The model under review builds one solid part; all positions refer to its coordinate system, in mm. Face numbers are marked on the shaded views. A direction names the side the tool comes from. Coordinates: 2 decimals unless noted, no trailing zeros. Order: outer loops, then holes, each group sorted by start corner. A loop starts at its lowest first (then second) coordinate and runs counter-clockwise, first axis right, second up. Notation, with made-up numbers: M 46.25,26 L 105.25,26 A13 ccw 105.25,33 Z; hole C 8,4 d7. An arc over 180 degrees is marked long. Answer as CSV lines item,"result". Start each with the question number.
Q1. Consider section C-C on z = 15. Write out the cut boundary in (x, y).
Q2. Consider section B-B on x = -29. Write out the cut boundary in (y, z), and give its area (3 significant figures).
Q3. Wall thickness on L1, parallel to Z at x = -2.95, y = -2.5; L2, parallel to Y at x = -29, z = 0; L3, parallel to X at y = -3, z = -17.5: over which ranges is each line inside the solid? List them lowest first. Write a range as [from, to].
Q4. Machinability: for the marked faces 4, 5 and 6, which of the approach directions +Z, -Z, +X, -X, +Y, -Y give a long, thin tool a straight path to every point of the face, cutting with its end or side? Answer none if there is none.
Q5. The part is to be moulded in two halves that separate along Y. For the marked faces 1, 2 and 3, say which applies: +Y half, -Y half, draft (parallel to the pull), parting line (faces both ways), or undercut.
Q6. Consider section A-A on z = -4.5. Write out the cut boundary in (x, y).
Q7. For P1, Ø0.9, axis at y = -6.5, z = -21, coming from the -X side; P2, Ø5, axis at x = -28.5, y = -3.5, coming from the -Z side; P3, Ø1.5, axis at x = -5.5, y = -5.5, coming from the -Z side; P4, Ø10.5, axis at y = -2.5, z = -15, coming from the +X side, all flat-tipped, find the tip position at first contact; note any pin that passes through.
Q8. Consider section D-D on y = -2.5. State how many separate pieces and enclosed holes the cut face has, and give its area (3 significant figures).
from build123d import *

# Parameters (mm, degrees)
F0_W          = 36.5
F0_H          = 20
F0_R          = 4.75
F1_DEPTH      = 5
F1_DEPTH_BACK = 5
F2_SIZE       = 2
F3_W          = 20
F3_H          = 46
F3_R          = 4
F4_DEPTH      = 4
F5_T4_DEPTH   = 20
F5_S5_R       = 4
F5_T6_DEPTH   = 16
F5_T10_DEPTH  = 20
F5_S11_R      = 4
F5_T12_DEPTH  = 16
F3_R_2        = 2.15
F6_DEPTH      = 4
F7_R          = 5
F8_R          = 5


# Not quite as in the source:
# - a fillet or chamfer that OpenCascade refuses, or shapes differently, is made with other operations: its cross-section is extruded or revolved along the edge and cut away or added


with BuildPart() as f1:
    # F0 (on Top) → F1 (new body, two sides)
    with BuildSketch(Plane.XY) as f1_sk:
        with Locations((-18.25, -2.5)):
            Rectangle(F0_W, F0_H)
        with Locations((-29, 0)):
            Circle(F0_R, mode=Mode.SUBTRACT)
    extrude(amount=F1_DEPTH)
    extrude(f1_sk.sketch, amount=-F1_DEPTH_BACK)

    # F2
    f2_edges = [f1.edges().sort_by_distance(p)[0] for p in [
        (-33.75, 0, 5),
        (-33.75, 0, -5),
    ]]
    chamfer(f2_edges, length=F2_SIZE)

    # F3 (on Right) → F4 (join)
    with BuildSketch(Plane.YZ):
        with Locations((-2.5, 0)):
            Rectangle(F3_W, F3_H)
        with Locations((-2.5, -15)):
            Circle(F3_R, mode=Mode.SUBTRACT)
        with Locations((-2.5, 15)):
            Circle(F3_R, mode=Mode.SUBTRACT)
    extrude(amount=-F4_DEPTH)

    # F5: fillet of radius 15 on 2 edges, made by hand


with BuildPart() as f5_tool2:
    # F5_s3 → F5_t4 (new body)
    with BuildSketch(Plane.XZ.offset(12.5)):
        with BuildLine():
            ThreePointArc((-19, 5), (-8.3933982822, 9.3933982822), (-4, 20))
            Line((-4, 20), (-4, 5))
            Line((-4, 5), (-19, 5))
        make_face()
    extrude(amount=-F5_T4_DEPTH)

    # F5_s5 → F5_t6 (cut, symmetric)
    with BuildSketch(Plane.YZ.offset(-11.5)):
        with Locations((-2.5, 15)):
            Circle(F5_S5_R)
    extrude(amount=F5_T6_DEPTH, both=True, mode=Mode.SUBTRACT)


with BuildPart() as f1_1:
    add(f1.part)

    # F5_t1: union F5_tool2
    add(f5_tool2.part)


with BuildPart() as f5_tool8:
    # F5_s9 → F5_t10 (new body)
    with BuildSketch(Plane.XZ.offset(12.5)):
        with BuildLine():
            ThreePointArc((-4, -20), (-8.3933982822, -9.3933982822), (-19, -5))
            Line((-19, -5), (-4, -5))
            Line((-4, -5), (-4, -20))
        make_face()
    extrude(amount=-F5_T10_DEPTH)

    # F5_s11 → F5_t12 (cut, symmetric)
    with BuildSketch(Plane.YZ.offset(-11.5)):
        with Locations((-2.5, -15)):
            Circle(F5_S11_R)
    extrude(amount=F5_T12_DEPTH, both=True, mode=Mode.SUBTRACT)


with BuildPart() as f1_2:
    add(f1_1.part)

    # F5_t7: union F5_tool8
    add(f5_tool8.part)

    # F3 (on Right) → F6 (join)
    with BuildSketch(Plane.YZ):
        with Locations((-2.5, 15)):
            Circle(F3_R)
        with Locations((-2.5, 15)):
            Circle(F3_R_2, mode=Mode.SUBTRACT)
        with Locations((-2.5, -15)):
            Circle(F3_R)
        with Locations((-2.5, -15)):
            Circle(F3_R_2, mode=Mode.SUBTRACT)
    extrude(amount=-F6_DEPTH)

    # F7
    f7_edges = [f1_2.edges().sort_by_distance(p)[0] for p in [
        (-2, -12.5, -23),
        (-2, -12.5, 23),
        (-2, 7.5, -23),
        (-2, 7.5, 23),
    ]]
    fillet(f7_edges, radius=F7_R)

    # F8
    f8_edges = [f1_2.edges().sort_by_distance(p)[0] for p in [
        (-36.5, -12.5, 0),
        (-36.5, 7.5, 0),
    ]]
    fillet(f8_edges, radius=F8_R)


solid = f1_2.part
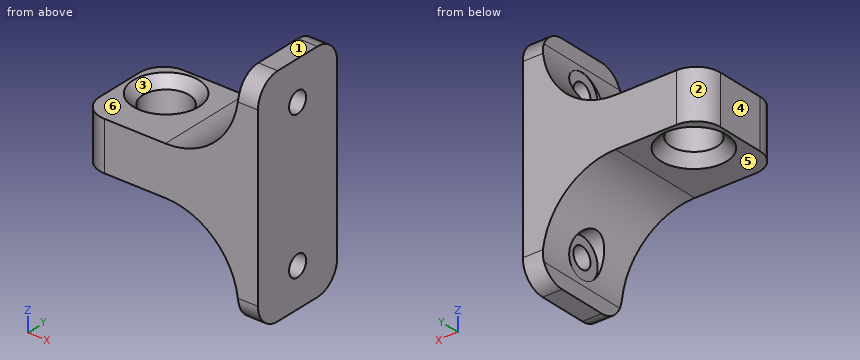
Evaluation:
1,outline,"M -4.86,-12.5 L 0,-12.5 L 0,-4.65 L -4,-4.65 L -4,-6.5 L -4.86,-6.5 Z; M -4.86,1.5 L -4,1.5 L -4,-0.35 L 0,-0.35 L 0,7.5 L -4.86,7.5 Z"
2,outline,"M -12.5,-5 L -6.75,-5 L -4.75,-3 L -4.75,3 L -6.75,5 L -12.5,5 Z; M 4.75,-3 L 6.75,-5 L 7.5,-5 L 7.5,5 L 6.75,5 L 4.75,3 Z"
2,area,"97.0 mm²"
3,L1,"z = [-23, -17.15], [-12.85, 12.85], [17.15, 23]"
3,L2,"y = [-12.5, -4.75], [4.75, 7.5]"
3,L3,"x = [-4, 0]"
4,face 4,"+Z, -Z, -X, +Y, -Y"
4,face 5,"-Z, -X, +Y, -Y"
4,face 6,"+Z, -X, +Y, -Y"
5,face 1,"draft"
5,face 2,"+Y half"
5,face 3,"undercut"
6,outline,"M -36.5,-7.5 A5 ccw -31.5,-12.5 L 0,-12.5 L 0,7.5 L -31.5,7.5 A5 ccw -36.5,2.5 Z; hole C -29,0 d12.5"
7,P1,"stops at x = -4"
7,P2,"stops at z = -4.29"
7,P3,"stops at z = -13.6"
7,P4,"stops at x = 0"
8,separate pieces,"4"
8,enclosed holes,"0"
8,area,"464 mm²"
